The model under review builds one solid part; all positions refer to its coordinate system, in mm. Face numbers are marked on the shaded views. A direction names the side the tool comes from. Coordinates: 2 decimals unless noted, no trailing zeros. Write each loop counter-clockwise with the first axis right and the second up, starting at its lowest first coordinate (ties: lowest second). Pieces come first, ordered by that corner, then holes. Notation, with made-up numbers: M 89.5,-34 L 146.5,-34 A14 cw 146.5,-28 Z; hole C 70,11 d7. An arc over 180 degrees is marked long. Answer as a JSON object with one key per item and string values.
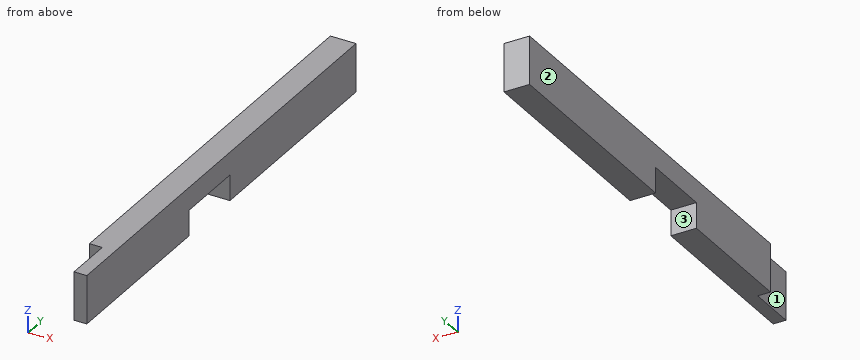
```python
from build123d import *

# Parameters (mm, degrees)
F0_W     = 36
F0_H     = 68
F1_DEPTH = 647
F2_W     = 98
F2_H     = 36
F3_DEPTH = 36
F5_W     = 68
F5_H     = 68
F6_DEPTH = 18


with BuildPart() as f1:
    # F0 (on Front) → F1 (new body)
    with BuildSketch(Plane.XZ):
        Rectangle(F0_W, F0_H)
    extrude(amount=F1_DEPTH)

    # F2 (on face) → F3 (cut, through all)
    with BuildSketch(Plane.YZ.offset(18)):
        with Locations((-352, -16)):
            Rectangle(F2_W, F2_H)
    extrude(amount=-F3_DEPTH, mode=Mode.SUBTRACT)

    # F5 (on face) → F6 (cut)
    with BuildSketch(Plane(origin=(-18, 0, 0), x_dir=(0, -1, 0), z_dir=(-1, 0, 0))):
        with Locations((613, 0)):
            Rectangle(F5_W, F5_H)
    extrude(amount=-F6_DEPTH, mode=Mode.SUBTRACT)


solid = f1.part
```
(1) For the marked faces 1, 2 and 3, list the 3-axis set-ups (+Z, -Z, +X, -X, +Y, -Y) from which the entire face can be reached by the end or side of a thin tool; tool diameter is ignored.
Results list:
{"face 1": "+Z, -Z, -X, -Y", "face 2": "+Z, -Z, -X, +Y, -Y", "face 3": "-Z, +X, -X"}
(2) Add section B-B on x = 7.5. Give the boundary of the cut face in (y, z), and give its area (3 significant figures).
Results list:
{"outline": "M -647,-34 L -401,-34 L -401,2 L -303,2 L -303,-34 L 0,-34 L 0,34 L -647,34 Z", "area": "40,500 mm²"}
(3) Add section A-A on z = -16. Give the boundary of the cut face in (x, y).
Results list:
{"outline": "M -18,-579 L 0,-579 L 0,-647 L 18,-647 L 18,-401 L -18,-401 Z; M -18,-303 L 18,-303 L 18,0 L -18,0 Z"}
(4) For pin 1 Ø10 at (x, y) = (-6, -360) entering from -Z; pin 2 Ø20.5 at (y, z) = (-603, -8) entering from -X; pin 3 Ø5.5 at (x, z) = (-12, 6) entering from -Y, all flat-tipped, find the tip position at first contact; note any pin that passes through.
Results list:
{"pin 1": "z = 2", "pin 2": "x = 0", "pin 3": "y = -579"}
(5) Add section C-C on z = 10.5. Give the boundary of the cut face in (x, y), and give its area (3 significant figures).
Results list:
{"outline": "M -18,-579 L 0,-579 L 0,-647 L 18,-647 L 18,0 L -18,0 Z", "area": "22,100 mm²"}
(6) Wall thickness on line 1 along Y through (x, z) = (-9, -8.5); line 2 along Y through (x, z) = (6.5, -19.5); line 3 along Z through (x, y) = (-9.5, -334): over which ranges is each line inside the solid? List them lowest first. Write a range as from..to.
Results list:
{"line 1": "-579..-401, -303..0", "line 2": "-647..-401, -303..0", "line 3": "2..34"}
